Model file for the job. Use its own axes, mm. Round coordinates to 2 decimals unless told otherwise and drop trailing zeros. Loops run counter-clockwise (first coordinate to the right, second up) from the corner with the lowest first, then second, coordinate; pieces in that order, holes last. Notation, with made-up numbers: (-31, 31) -> (18, 31) arc R21 ccw to (18, 49) -> close; hole circle Ø3 at (10, 9). An arc over 180 degrees is marked (long way). Use a Markdown table: item, result.
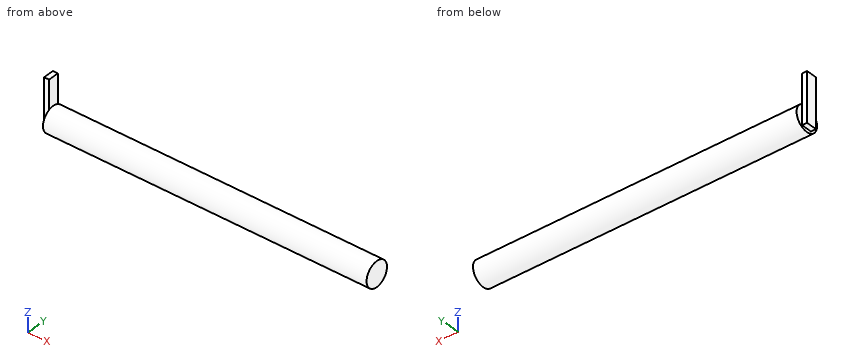
from build123d import *

# Parameters (mm, degrees)
F0_R     = 3.175
F1_DEPTH = 82.55
F2_W     = 2.726714
F2_H     = 1.16385
F3_DEPTH = 1.27
F4_W     = 1.27
F4_H     = 2.726714
F5_DEPTH = 7.62
F6_W     = 1.27
F6_H     = 2.726714
F7_DEPTH = 3.81


with BuildPart() as f1:
    # F0 (on Right) → F1 (new body)
    with BuildSketch(Plane.YZ):
        Circle(F0_R)
    extrude(amount=F1_DEPTH)

    # F2 (on face) → F3 (join)
    with BuildSketch(Plane.YZ):
        with Locations((0.08243, 2.065926)):
            Rectangle(F2_W, F2_H)
    extrude(amount=-F3_DEPTH)

    # F4 (on face) → F5 (join)
    with BuildSketch(Plane.XY.offset(2.647851)):
        with Locations((-0.635, 0.08243)):
            Rectangle(F4_W, F4_H)
    extrude(amount=F5_DEPTH)

    # F6 (on face) → F7 (join)
    with BuildSketch(Plane(origin=(0, 0, 1.484001), x_dir=(1, 0, 0), z_dir=(0, 0, -1))):
        with Locations((-0.635, -0.08243)):
            Rectangle(F6_W, F6_H)
    extrude(amount=F7_DEPTH)


solid = f1.part
Q1. Drill centre lines: L1, parallel to Y at x = 35.5, z = 0.25; L2, parallel to X at y = 1, z = 7.5; L3, parallel to X at y = 1.75, z = -1. Where is each one in solid material? Low to high. Write a range as from..to.
Results list:
| item | result |
|---|---|
| L1 | y = -3.17..3.17 |
| L2 | x = -1.27..0 |
| L3 | x = 0..82.55 |
Q2. Flat gauge pins, fed straight in: pin 1 (0.8 mm diameter, centred on y = -0.5, z = 5.5, fed in from +X); pin 2 (1.4 mm diameter, centred on x = -0.5, z = 3, fed in from -Y); pin 3 (1.4 mm diameter, centred on x = -0.5, z = 6, fed in from +Y). Where does each tip first touch, or does it go through?
Results list:
| item | result |
|---|---|
| pin 1 | stops at x = 0 |
| pin 2 | stops at y = -1.94 |
| pin 3 | stops at y = 1.45 |
Q3. Band-saw the part on C-C, the plane x = 18. Give the cut face in (y, z) (3 decimals).
Results list:
| item | result |
|---|---|
| outline | circle Ø6.35 at (0, 0) |
Q4. Band-saw the part on D-D, the plane z = 6. Give the cut face in (x, y).
Results list:
| item | result |
|---|---|
| outline | (-1.27, -1.28) -> (0, -1.28) -> (0, 1.45) -> (-1.27, 1.45) -> close |
Q5. Band-saw the part on B-B, the plane z = -1.5. Give the cut face in (x, y).
Results list:
| item | result |
|---|---|
| outline | (-1.27, -1.28) -> (0, -1.28) -> (0, -2.8) -> (82.55, -2.8) -> (82.55, 2.8) -> (0, 2.8) -> (0, 1.45) -> (-1.27, 1.45) -> close |
Q6. Band-saw the part on A-A, the plane y = 0. Give the cut face in (x, z) (3 decimals), plus the area to 3 significant figures.
Results list:
| item | result |
|---|---|
| outline | (-1.27, -2.326) -> (0, -2.326) -> (0, -3.175) -> (82.55, -3.175) -> (82.55, 3.175) -> (0, 3.175) -> (0, 10.268) -> (-1.27, 10.268) -> close |
| area | 540 mm² |
